For this review, take the finished solid that the model builds, in its own axes (mm). Face numbers are marked on the shaded views. Give positions to 0.01 mm unless a question says otherwise; leave off trailing zeros. Write each loop counter-clockwise with the first axis right and the second up, starting at its lowest first coordinate (ties: lowest second). Pieces come first, ordered by that corner, then holes.
1) We need section B-B on z = 59.5. Give the boundary of the cut face in (x, y), and give its area (3 significant figures).
2) For P1, Ø8, axis at y = 8.5, z = 35.5, coming from the +X side; P2, Ø4, axis at y = -10, z = 51, coming from the -X side; P3, Ø8, axis at y = -5.5, z = 39.5, coming from the +X side, all flat-tipped, find the tip position at first contact; note any pin that passes through.
3) Wall thickness on line 1 along Z through (x, y) = (0, 5); line 2 along Z through (x, y) = (-3.25, -1); line 3 along X through (y, z) = (6, 53): over which ranges is each line inside the solid? List them lowest first.
4) Draft analysis for pull direction Z (two halves, no side actions). For the marked faces 1, 2 and 3, state which applies: pulls with the +Z half, pulls with the -Z half, needs draft (parallel to the pull), parting line crosses it, or undercut.
5) We need section A-A on x = 0. Give the boundary of the cut face in (y, z), and give its area (3 significant figures).
6) We need section D-D on x = -9.25. Give the boundary of the cut face in (y, z), and give its area (3 significant figures).
7) We need section C-C on y = -3. Give the boundary of the cut face in (x, z).
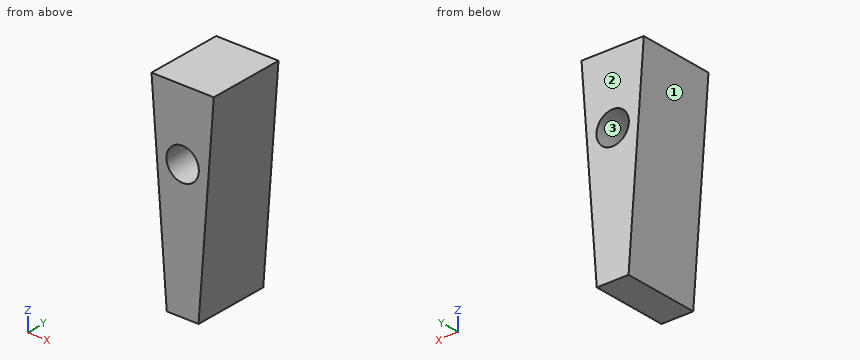
from build123d import *

# Parameters (mm, degrees)
F0_W     = 25
F0_H     = 31
F1_DEPTH = 86.3
F2_R     = 6.5
F3_DEPTH = 31.5
F5_DEPTH = 31.001
F6_W     = 20
F6_H     = 5
F7_DEPTH = 50


with BuildPart() as f1:
    # F0 (on Top) → F1 (new body)
    with BuildSketch(Plane.XY):
        Rectangle(F0_W, F0_H)
    extrude(amount=F1_DEPTH)

    # F2 (on Front) → F3 (cut, symmetric)
    with BuildSketch(Plane.XZ):
        with Locations((0, 58.577)):
            Circle(F2_R)
    extrude(amount=F3_DEPTH, both=True, mode=Mode.SUBTRACT)

    # F4 (on face) → F5 (cut, through all)
    with BuildSketch(Plane(origin=(0, 15.5, 0), x_dir=(-1, 0, 0), z_dir=(0, 1, 0))):
        Polygon((12.5, 0), (12.5, 86.3), (6, 0), align=None)
        Polygon((-6, 0), (-12.5, 86.3), (-12.5, 0), align=None)
    extrude(amount=-F5_DEPTH, mode=Mode.SUBTRACT)

    # F6 (on Front) → F7 (cut, symmetric)
    with BuildSketch(Plane.XZ):
        with Locations((0, 2.5)):
            Rectangle(F6_W, F6_H)
    extrude(amount=F7_DEPTH, both=True, mode=Mode.SUBTRACT)


solid = f1.part
Results list:
1. outline: (-10.48, -15.5) - (-6.43, -15.5) - (-6.43, 15.5) - (-10.48, 15.5) - close; (6.43, -15.5) - (10.48, -15.5) - (10.48, 15.5) - (6.43, 15.5) - close
1. area: 251 mm2
2. P1: stops at x = 8.98
2. P2: stops at x = -9.99
2. P3: stops at x = 9.28
3. line 1: z = 5 to 52.08, 65.08 to 86.3
3. line 2: z = 5 to 52.95, 64.21 to 86.3
3. line 3: x = -9.99 to -3.34, 3.34 to 9.99
4. face 1: pulls with the -Z half
4. face 2: needs draft
4. face 3: undercut
5. outline: (-15.5, 5) - (15.5, 5) - (15.5, 52.08) - (-15.5, 52.08) - close; (-15.5, 65.08) - (15.5, 65.08) - (15.5, 86.3) - (-15.5, 86.3) - close
5. area: 2,120 mm2
6. outline: (-15.5, 43.15) - (15.5, 43.15) - (15.5, 86.3) - (-15.5, 86.3) - close
6. area: 1,340 mm2
7. outline: (-12.5, 86.3) - (-6.38, 5) - (6.38, 5) - (12.5, 86.3) - close; hole circle Ø13 at (0, 58.58)
